Study the drawing (mm; zero at the part's minimum x, y, z) and answer. Round coordinates to 2 decimals unless told otherwise and drop trailing zeros. Loops run counter-clockwise (first coordinate to the right, second up) from the corner with the lowest first, then second, coordinate; pieces in that order, holes last. Notation, with made-up numbers: M 47,82.5 L 86,82.5 A13 cw 86,106.5 Z; hole C -0.5,9.5 d7. An arc over 180 degrees is marked long. Write each question's results on one line, items separated by ' | '.
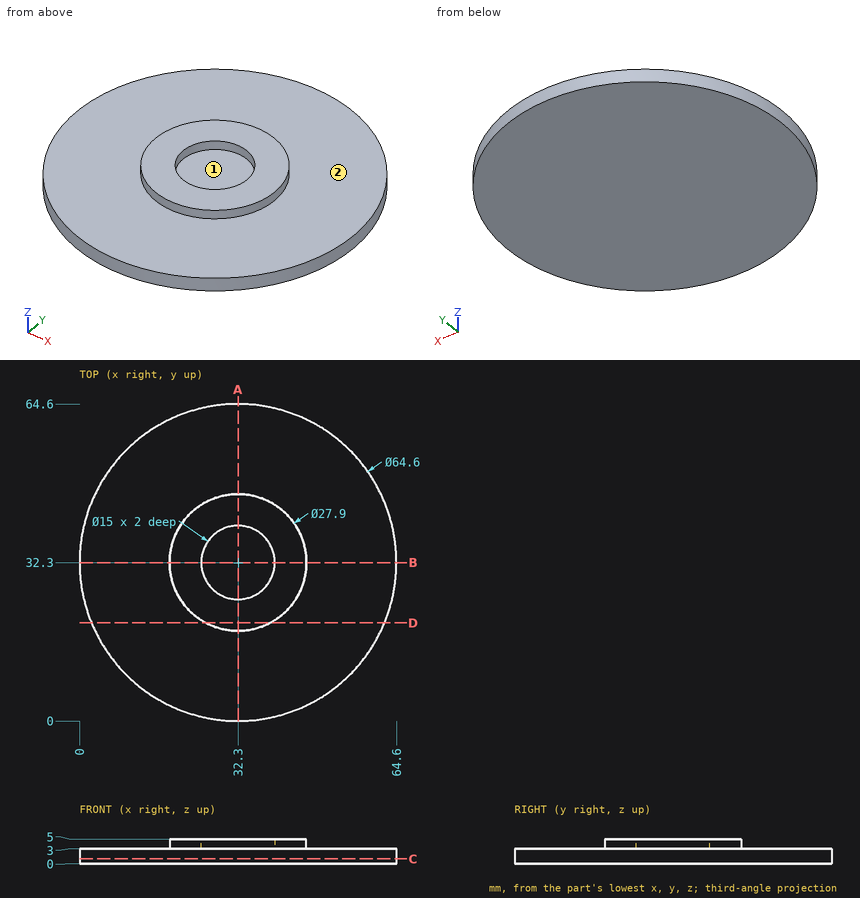
Item 1: The part is cut by section A-A (x = 32.3). Determine the outline of the cut face in (y, z).
Outcome:
outline: M 0,0 L 64.6,0 L 64.6,3 L 46.25,3 L 46.25,5 L 39.8,5 L 39.8,3 L 24.8,3 L 24.8,5 L 18.35,5 L 18.35,3 L 0,3 Z
Item 2: Straight lines are drawn through the part: line 1 (Y direction, x = 32.3, z = 3.7); line 2 (Z direction, x = 17, y = 36); line 3 (Y direction, x = 17.5, z = 0.9). For each, find the intervals that lie inside material, in ascending order.
Outcome:
line 1: y = 18.35 to 24.8, 39.8 to 46.25 | line 2: z = 0 to 3 | line 3: y = 3.59 to 61.01
Item 3: The part is cut by section D-D (y = 20). Determine the outline of the cut face in (x, z).
Outcome:
outline: M 2.43,0 L 62.17,0 L 62.17,3 L 38.88,3 L 38.88,5 L 25.72,5 L 25.72,3 L 2.43,3 Z
Item 4: The part is cut by section C-C (z = 0.95). Determine the outline of the cut face in (x, y).
Outcome:
outline: C 32.3,32.3 d64.6
Item 5: Flat-ended cylindrical pins translate along their axes: pin 1 (10 mm diameter, centred on x = 52.5, y = 38, fed in from +Z); pin 2 (19.5 mm diameter, centred on x = 46.5, y = 23.5, fed in from +Z). Find the tip coordinate at first contact, or state that the pin passes through.
Outcome:
pin 1: stops at z = 3 | pin 2: stops at z = 5
Item 6: The mould has two halves that part along X. Classify the marked faces 1 and 2: pulls with the +X half, pulls with the -X half, needs draft (parallel to the pull), parting line crosses it, or undercut.
Outcome:
face 1: undercut | face 2: needs draft
